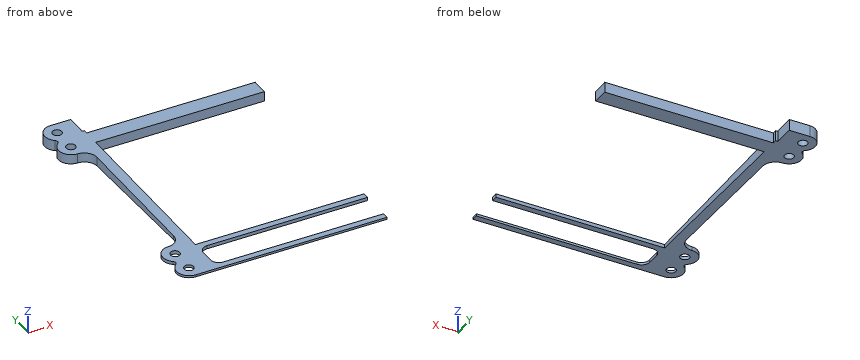
from build123d import *

# Parameters (mm, degrees)
BOSS_EXTRUDE1_OUTLINE_R = 3.556
BOSS_EXTRUDE1_OUTLINE_W = 260.9469
BOSS_EXTRUDE1_OUTLINE_H = 138.1252
BOSS_EXTRUDE1_DEPTH     = 76.2
CUT_EXTRUDE1_DEPTH      = 355.32482824
CUT_EXTRUDE1_DEPTH_BACK = 355.32482824
FILLET1_R               = 2.54
SKETCH7_W               = 260.9469
SKETCH7_H               = 22.1996
CUT_EXTRUDE2_DEPTH      = 347.152897849
FILLET2_R               = 6.35
SKETCH8_W               = 217.439036591
SKETCH8_H               = 235.521960295
CUT_EXTRUDE4_DEPTH      = 347.144751077


# Read off the part's stored shape, not the designer's step: Boss-Extrude1
with BuildPart() as part:
    # Boss-Extrude1 outline → Boss-Extrude1 (new body)
    with BuildSketch(Plane.XY):
        with BuildLine():
            Line((-286.3596, -22.225), (9.525, -22.225))
            ThreePointArc((9.525, -22.225), (19.05, -12.7), (9.525, -3.175))
            ThreePointArc((9.525, -3.175), (19.05, 6.35), (9.525, 15.875))
            ThreePointArc((9.525, 15.875), (2.789807909, 18.664807909), (0, 25.4))
            Line((0, 25.4), (0, 131.7752))
            ThreePointArc((0, 131.7752), (2.789807909, 138.510392091), (9.525, 141.3002))
            ThreePointArc((9.525, 141.3002), (19.05, 150.8252), (9.525, 160.3502))
            ThreePointArc((9.525, 160.3502), (19.05, 169.8752), (9.525, 179.4002))
            Line((9.525, 179.4002), (-6.35, 179.4002))
            Line((-6.35, 179.4002), (-6.35, 163.5252))
            Line((-6.35, 163.5252), (-7.9502, 163.5252))
            Line((-7.9502, 163.5252), (-7.9502, 160.3502))
            Line((-7.9502, 160.3502), (-268.9098, 160.3502))
            Line((-268.9098, 160.3502), (-268.9098, 163.5252))
            Line((-268.9098, 163.5252), (-270.51, 163.5252))
            Line((-270.51, 163.5252), (-270.51, 179.4002))
            Line((-270.51, 179.4002), (-286.385, 179.4002))
            ThreePointArc((-286.385, 179.4002), (-295.91, 169.8752), (-286.385, 160.3502))
            ThreePointArc((-286.385, 160.3502), (-295.897297883, 150.818850004), (-286.3723, 141.3002))
            ThreePointArc((-286.3723, 141.3002), (-279.637107909, 138.510392091), (-276.8473, 131.7752))
            Line((-276.8473, 131.7752), (-276.8473, 25.4))
            ThreePointArc((-276.8473, 25.4), (-279.637107909, 18.664807909), (-286.3723, 15.875))
            ThreePointArc((-286.3723, 15.875), (-295.8973, 6.35), (-286.3723, -3.175))
            ThreePointArc((-286.3723, -3.175), (-295.884597883, -12.706349996), (-286.3596, -22.225))
        make_face()
        with Locations((-286.3596, -12.7)):
            Circle(BOSS_EXTRUDE1_OUTLINE_R, mode=Mode.SUBTRACT)
        with Locations((-286.3723, 6.35)):
            Circle(BOSS_EXTRUDE1_OUTLINE_R, mode=Mode.SUBTRACT)
        with Locations((9.525, -12.7)):
            Circle(BOSS_EXTRUDE1_OUTLINE_R, mode=Mode.SUBTRACT)
        with Locations((9.525, 6.35)):
            Circle(BOSS_EXTRUDE1_OUTLINE_R, mode=Mode.SUBTRACT)
        with Locations((-286.3723, 150.8252)):
            Circle(BOSS_EXTRUDE1_OUTLINE_R, mode=Mode.SUBTRACT)
        with Locations((-286.385, 169.8752)):
            Circle(BOSS_EXTRUDE1_OUTLINE_R, mode=Mode.SUBTRACT)
        with Locations((-138.42365, 78.5876)):
            Rectangle(BOSS_EXTRUDE1_OUTLINE_W, BOSS_EXTRUDE1_OUTLINE_H, mode=Mode.SUBTRACT)
        with Locations((9.525, 150.8252)):
            Circle(BOSS_EXTRUDE1_OUTLINE_R, mode=Mode.SUBTRACT)
        with Locations((9.525, 169.8752)):
            Circle(BOSS_EXTRUDE1_OUTLINE_R, mode=Mode.SUBTRACT)
    extrude(amount=BOSS_EXTRUDE1_DEPTH)

    # Sketch5 → Cut-Extrude1 (cut, two sides: drawn at the far end of the back side and taken through both)
    with BuildSketch(Plane.ZY.offset(276.8473).offset(-CUT_EXTRUDE1_DEPTH_BACK)):
        Polygon((1.6002, -22.225), (8.641107133, 179.4002), (76.2, 179.4002), (76.2, -22.225), align=None)
    extrude(amount=CUT_EXTRUDE1_DEPTH + CUT_EXTRUDE1_DEPTH_BACK, mode=Mode.SUBTRACT)

    # Fillet1
    fillet1_edges = [part.edges().sort_by_distance(p)[0] for p in [
        (-286.385, 160.3502, 3.987933237),
        (-286.3723, -3.175, 1.132720329),
        (9.525, -3.175, 1.132720329),
        (9.525, 160.3502, 3.987933237),
    ]]
    fillet(fillet1_edges, radius=FILLET1_R)

    # Sketch7 → Cut-Extrude2 (cut, through all)
    with BuildSketch(Plane(origin=(0, 0, 0), x_dir=(-1, 0, 0), z_dir=(0, 0, -1))):
        with Locations((138.42365, -6.35)):
            Rectangle(SKETCH7_W, SKETCH7_H)
    extrude(amount=-CUT_EXTRUDE2_DEPTH, mode=Mode.SUBTRACT)

    # Fillet2
    fillet2_edges = [part.edges().sort_by_distance(p)[0] for p in [
        (-268.8971, 4.7498, 1.271090386),
        (-268.8971, -17.4498, 0.883476829),
        (-7.9502, -17.4498, 0.883476829),
        (-7.9502, 4.7498, 1.271090386),
    ]]
    fillet(fillet2_edges, radius=FILLET2_R)

    # Sketch8 → Cut-Extrude4 (cut, through all)
    with BuildSketch(Plane(origin=(0, -0.082881646, 2.373419811), x_dir=(1, 0, 0), z_dir=(0, -0.03489949670250444, 0.9993908270190958))):
        with Locations((-29.704131704, 74.917246318)):
            Rectangle(SKETCH8_W, SKETCH8_H)
    extrude(amount=-CUT_EXTRUDE4_DEPTH, mode=Mode.SUBTRACT)


solid = part.part
Geometry: final body of the model. Coordinates: model frame, mm. Round coordinates to 2 decimals unless told otherwise and drop trailing zeros. Order: outer loops, then holes, each group sorted by start corner. A loop starts at its lowest first (then second) coordinate and runs counter-clockwise, first axis right, second up. Notation, with made-up numbers: (23, 82.5) -> (68, 82.5) arc R30 ccw to (68, 106.5) -> close; hole circle Ø1 at (-15.75, 43). An arc over 180 degrees is marked (long way). Put each result on its own line as item: value. Start each with the question number.
Q1. Section A-A on x = -172. Return the cut outline in (y, z) (3 decimals).
Q2. Section C-C on y = 32.5. Return the cut outline in (x, z).
Q3. Line query: probe 1 along Y at (x, z) = (-285.5, 6.5); probe 2 along Y at (x, z) = (-169, 7); probe 3 along Z at (x, y) = (-219, 155). Output: solid intervals per line, ascending.
Q4. Section B-B on y = 137.5. Return the cut outline in (x, z), and give its area (3 significant figures).
Q5. First-contact query: pin 1 (4.5 mm diameter, centred on x = -286.38, y = 169.88, fed in from +Z); pin 2 (2.5 mm diameter, centred on y = 78, z = 4.5, fed in from +X); pin 3 (1.5 mm diameter, centred on x = -188.5, z = 1.5, fed in from +Y); pin 4 (2 mm diameter, centred on y = 91, z = 3, fed in from -X). Flat tips, straight axial feed; report the tip coordinate or a pass-through.
Ans:
1. outline: (-22.225, 0) -> (-17.45, 0) -> (-17.45, 1.767) -> (-22.225, 1.6) -> close; (4.75, 0) -> (9.525, 0) -> (9.525, 2.709) -> (4.75, 2.542) -> close; (147.65, 0) -> (160.35, 0) -> (160.35, 7.976) -> (147.65, 7.532) -> close
2. outline: (-276.85, 0) -> (-268.9, 0) -> (-268.9, 3.51) -> (-276.85, 3.51) -> close
3. probe 1: y = 141.26 to 147.38, 154.27 to 166.43, 173.32 to 179.4
3. probe 2: y = 147.65 to 160.35
3. probe 3: z = 0 to 7.79
4. outline: (-278.76, 0) -> (-268.9, 0) -> (-268.9, 7.18) -> (-278.76, 7.18) -> close
4. area: 70.8 mm2
5. pin 1: passes through
5. pin 2: stops at x = -268.9
5. pin 3: stops at y = 160.35
5. pin 4: stops at x = -276.85
